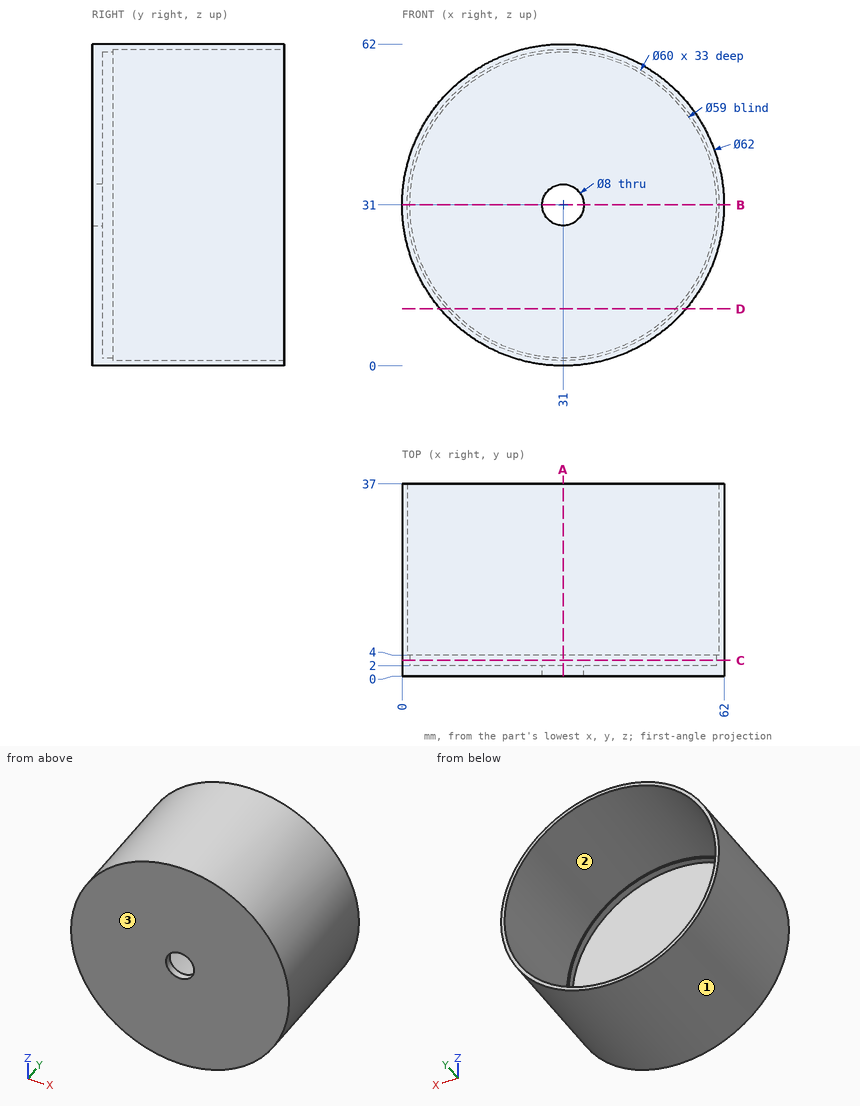
Input: dimensioned drawing with shaded views. Units: mm. Origin: part minimum x, y, z. Round coordinates to 2 decimals unless told otherwise and drop trailing zeros. Loops run counter-clockwise (first coordinate to the right, second up) from the corner with the lowest first, then second, coordinate; pieces in that order, holes last. Notation, with made-up numbers: (11, 29) -> (23, 29) arc R20 ccw to (23, 66) -> close; hole circle Ø1 at (38, -15.75). An arc over 180 degrees is marked (long way). Use one line per item in the form item = value. Start each with the question number.
1) Section D-D on z = 11. Output: boundary loops of the cut face in (x, y).
2) First-contact query: P1, Ø3, axis at x = 29, y = 28.5, coming from the +Z side; P2, Ø1.5, axis at y = 26.5, z = 51.5, coming from the -X side; P3, Ø6, axis at y = 10, z = 48, coming from the -X side. Flat tips, straight axial feed; report the tip coordinate or a pass-through.
3) Section A-A on x = 31. Output: boundary loops of the cut face in (y, z).
4) Draft query along Z for the marked faces 1, 2 and 3. Return one class per face: released by +Z, released by -Z, zero draft, split by the parting line, or undercut.
5) Line query: L1, parallel to X at y = 1.45, z = 31; L2, parallel to Z at x = 31.5, y = 28.5; L3, parallel to X at y = 3, z = 31. Output: solid intervals per line, ascending.
6) Section B-B on z = 31. Output: boundary loops of the cut face in (x, y), then the cut area to 3 significant figures.
7) Section C-C on y = 3. Output: boundary loops of the cut face in (x, z).
Response:
q1.outline = (7.31, 0) -> (54.69, 0) -> (54.69, 37) -> (53.36, 37) -> (53.36, 4) -> (52.69, 4) -> (52.69, 2) -> (9.31, 2) -> (9.31, 4) -> (8.64, 4) -> (8.64, 37) -> (7.31, 37) -> close
q2.P1 = 62
q2.P2 = 7.11
q2.P3 = 3.34
q3.outline = (0, 0) -> (37, 0) -> (37, 1) -> (4, 1) -> (4, 1.5) -> (2, 1.5) -> (2, 27) -> (0, 27) -> close; (0, 35) -> (2, 35) -> (2, 60.5) -> (4, 60.5) -> (4, 61) -> (37, 61) -> (37, 62) -> (0, 62) -> close
q4.face_1 = split by the parting line
q4.face_2 = undercut
q4.face_3 = zero draft
q5.L1 = 0 to 27, 35 to 62
q5.L2 = 0 to 1, 61 to 62
q5.L3 = 0 to 1.5, 60.5 to 62
q6.outline = (0, 0) -> (27, 0) -> (27, 2) -> (1.5, 2) -> (1.5, 4) -> (1, 4) -> (1, 37) -> (0, 37) -> close; (35, 0) -> (62, 0) -> (62, 37) -> (61, 37) -> (61, 4) -> (60.5, 4) -> (60.5, 2) -> (35, 2) -> close
q6.area = 180 mm^2
q7.outline = circle Ø62 at (31, 31); hole circle Ø59 at (31, 31)
